Build history of the part. All positions in model axes, mm. Round coordinates to 2 decimals unless told otherwise and drop trailing zeros. Order: outer loops, then holes, each group sorted by start corner. A loop starts at its lowest first (then second) coordinate and runs counter-clockwise, first axis right, second up. Notation, with made-up numbers: (45.25, -10) -> (95.25, -10) arc R9 cw to (95.25, 1) -> close; hole circle Ø7 at (-10.5, 84.5). An arc over 180 degrees is marked (long way). Write item = value, one per line.
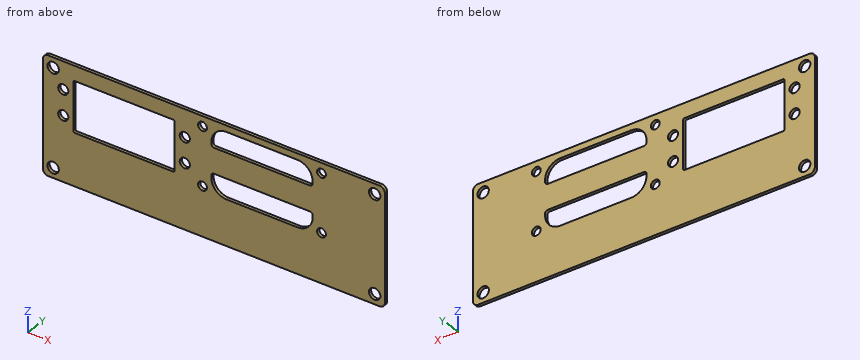
from build123d import *

# Parameters (mm, degrees)
BASE_R      = 2.25
BASE_R_2    = 1.75
BASE_R_3    = 2
SHEET_DEPTH = 1.2192


with BuildPart() as part:
    # BASE → SHEET (new body)
    with BuildSketch(Plane(origin=(0, 0, 0), x_dir=(1, 0, 0), z_dir=(0, 1, 0))):
        with BuildLine():
            Line((65.5, -23.25), (-65.5, -23.25))
            ThreePointArc((-65.5, -23.25), (-66.914213562, -22.664213562), (-67.5, -21.25))
            Line((-67.5, -21.25), (-67.5, 21.25))
            ThreePointArc((-67.5, 21.25), (-66.914213562, 22.664213562), (-65.5, 23.25))
            Line((-65.5, 23.25), (65.5, 23.25))
            ThreePointArc((65.5, 23.25), (66.914213562, 22.664213562), (67.5, 21.25))
            Line((67.5, 21.25), (67.5, -21.25))
            ThreePointArc((67.5, -21.25), (66.914213562, -22.664213562), (65.5, -23.25))
        make_face()
        with Locations(Location((-63.5, 19.25, 0), (0, 0, 270))):
            Circle(BASE_R, mode=Mode.SUBTRACT)
        with Locations(Location((-63.5, -19.25, 0), (0, 0, 270))):
            Circle(BASE_R, mode=Mode.SUBTRACT)
        with Locations(Location((63.5, -19.25, 0), (0, 0, 270))):
            Circle(BASE_R, mode=Mode.SUBTRACT)
        with Locations(Location((63.5, 19.25, 0), (0, 0, 270))):
            Circle(BASE_R, mode=Mode.SUBTRACT)
        with Locations(Location((-4.5, 3.75, 0), (0, 0, 270))):
            Circle(BASE_R_2, mode=Mode.SUBTRACT)
        with Locations(Location((42.5, 3.75, 0), (0, 0, 270))):
            Circle(BASE_R_2, mode=Mode.SUBTRACT)
        with Locations(Location((42.5, -19.25, 0), (0, 0, 270))):
            Circle(BASE_R_2, mode=Mode.SUBTRACT)
        with Locations(Location((-4.5, -19.25, 0), (0, 0, 270))):
            Circle(BASE_R_2, mode=Mode.SUBTRACT)
        with Locations(Location((-59.5, -2.4, 0), (0, 0, 270))):
            Circle(BASE_R_3, mode=Mode.SUBTRACT)
        with Locations(Location((-59.5, -12.4, 0), (0, 0, 270))):
            Circle(BASE_R_3, mode=Mode.SUBTRACT)
        with Locations(Location((-11.5, -2.4, 0), (0, 0, 270))):
            Circle(BASE_R_3, mode=Mode.SUBTRACT)
        with Locations(Location((-11.5, -12.4, 0), (0, 0, 270))):
            Circle(BASE_R_3, mode=Mode.SUBTRACT)
        with BuildLine():
            Line((5, -20.75), (33, -20.75))
            ThreePointArc((33, -20.75), (37.242640687, -18.992640687), (39, -14.75))
            Line((39, -14.75), (39, -13.75))
            ThreePointArc((39, -13.75), (38.707106781, -13.042893219), (38, -12.75))
            Line((38, -12.75), (0, -12.75))
            ThreePointArc((0, -12.75), (-0.707106781, -13.042893219), (-1, -13.75))
            Line((-1, -13.75), (-1, -14.75))
            ThreePointArc((-1, -14.75), (0.757359313, -18.992640687), (5, -20.75))
        make_face(mode=Mode.SUBTRACT)
        with BuildLine():
            Line((5, 5.25), (33, 5.25))
            ThreePointArc((33, 5.25), (37.242640687, 3.492640687), (39, -0.75))
            Line((39, -0.75), (39, -1.75))
            ThreePointArc((39, -1.75), (38.707106781, -2.457106781), (38, -2.75))
            Line((38, -2.75), (0, -2.75))
            ThreePointArc((0, -2.75), (-0.707106781, -2.457106781), (-1, -1.75))
            Line((-1, -1.75), (-1, -0.75))
            ThreePointArc((-1, -0.75), (0.757359313, 3.492640687), (5, 5.25))
        make_face(mode=Mode.SUBTRACT)
        with BuildLine():
            Line((-55, -17.4), (-16, -17.4))
            ThreePointArc((-16, -17.4), (-15.646446609, -17.253553391), (-15.5, -16.9))
            Line((-15.5, -16.9), (-15.5, 2.1))
            ThreePointArc((-15.5, 2.1), (-15.646446609, 2.453553391), (-16, 2.6))
            Line((-16, 2.6), (-55, 2.6))
            ThreePointArc((-55, 2.6), (-55.353553391, 2.453553391), (-55.5, 2.1))
            Line((-55.5, 2.1), (-55.5, -16.9))
            ThreePointArc((-55.5, -16.9), (-55.353553391, -17.253553391), (-55, -17.4))
        make_face(mode=Mode.SUBTRACT)
    extrude(amount=SHEET_DEPTH)


solid = part.part
Q1. Cut at A-A, the plane x = -4.5. List the corners of the cut face in (y, z), and give its area (3 significant figures).
Check values:
outline = (0, -23.25) -> (1.22, -23.25) -> (1.22, -5.5) -> (0, -5.5) -> close; (0, -2) -> (1.22, -2) -> (1.22, 17.5) -> (0, 17.5) -> close; (0, 21) -> (1.22, 21) -> (1.22, 23.25) -> (0, 23.25) -> close
area = 48.2 mm²
Q2. Cut at B-B, the plane z = -19.25. List the corners of the cut face in (x, y).
Check values:
outline = (-67.5, 0) -> (-65.75, 0) -> (-65.75, 1.22) -> (-67.5, 1.22) -> close; (-61.25, 0) -> (61.25, 0) -> (61.25, 1.22) -> (-61.25, 1.22) -> close; (65.75, 0) -> (67.5, 0) -> (67.5, 1.22) -> (65.75, 1.22) -> close
Q3. Cut at C-C, the plane x = -52. List the corners of the cut face in (y, z), and give its area (3 significant figures).
Check values:
outline = (0, -23.25) -> (1.22, -23.25) -> (1.22, -2.6) -> (0, -2.6) -> close; (0, 17.4) -> (1.22, 17.4) -> (1.22, 23.25) -> (0, 23.25) -> close
area = 32.3 mm²
Q4. Cut at D-D, the plane z = -3.75. List the corners of the cut face in (x, y).
Check values:
outline = (-67.5, 0) -> (-6.25, 0) -> (-6.25, 1.22) -> (-67.5, 1.22) -> close; (-2.75, 0) -> (1.03, 0) -> (1.03, 1.22) -> (-2.75, 1.22) -> close; (36.97, 0) -> (40.75, 0) -> (40.75, 1.22) -> (36.97, 1.22) -> close; (44.25, 0) -> (67.5, 0) -> (67.5, 1.22) -> (44.25, 1.22) -> close
Q5. Probe probe 1 along X at (y, z) = (0.35, -19.25); probe 2 along Z at (x, y) = (10.5, 0.7); probe 3 along Z at (x, y) = (-16, 0.9). List the from-to ranges inside material, lowest first.
Check values:
probe_1 = -67.5 to -65.75, -61.25 to 61.25, 65.75 to 67.5
probe_2 = -23.25 to -5.25, 2.75 to 12.75, 20.75 to 23.25
probe_3 = -23.25 to -2.6, 17.4 to 23.25
Q6. Flat gauge pin, fed straight in: pin 1 (3 mm diameter, centred on x = -4.5, z = 19.25, fed in from +Y). Where does the tip first touch, or does it go through?
Check values:
pin_1 = through
